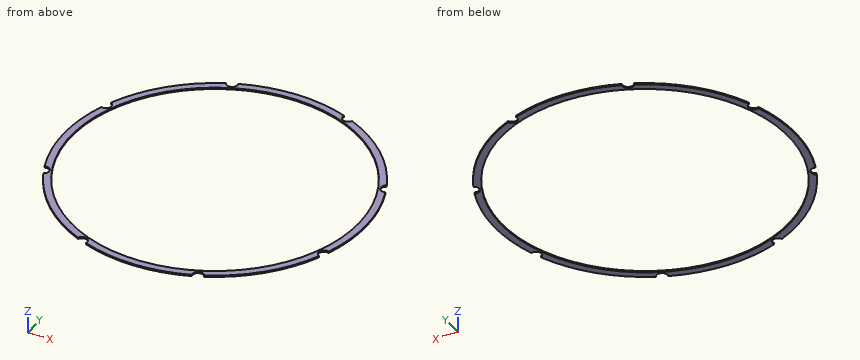
```python
from build123d import *

# Parameters (mm, degrees)
CYLINDER1506_R               = 1.5
CYLINDER1506_DEPTH           = 32
CYLINDER1506_PLACEMENT_ANGLE = 45
CYLINDER1509_R               = 1.5
CYLINDER1509_DEPTH           = 32
CYLINDER1510_R               = 1.5
CYLINDER1510_DEPTH           = 32
CYLINDER1510_PLACEMENT_ANGLE = 135
CYLINDER1511_R               = 1.5
CYLINDER1511_DEPTH           = 32
CYLINDER1508_R               = 1.5
CYLINDER1508_DEPTH           = 32
CYLINDER1508_PLACEMENT_ANGLE = 225
CYLINDER1512_R               = 1.5
CYLINDER1512_DEPTH           = 32
CYLINDER1505_R               = 1.5
CYLINDER1505_DEPTH           = 32
CYLINDER1505_PLACEMENT_ANGLE = 45
CYLINDER1504_R               = 1.5
CYLINDER1504_DEPTH           = 32
COMPOUND1000_PLACEMENT_ANGLE = 22.5
TUBE139_R                    = 42
TUBE139_R_2                  = 40
TUBE139_DEPTH                = 0.4


with BuildPart() as obj1:
    # Cylinder1506 → Cylinder1506 (new body)
    with BuildSketch(Plane.XY):
        Circle(CYLINDER1506_R)
    extrude(amount=CYLINDER1506_DEPTH)


with BuildPart() as obj1_1:
    # Cylinder1506 placement: moved
    add(obj1.part.moved(Location((29.698485, -29.698485, 33.5))).rotate(Axis((29.698485, -29.698485, 33.5), (0, 0, 1)), CYLINDER1506_PLACEMENT_ANGLE))


with BuildPart() as obj2:
    # Cylinder1509 → Cylinder1509 (new body)
    with BuildSketch(Plane(origin=(42, 0, 33.5), x_dir=(0, 1, 0), z_dir=(0, 0, 1))):
        Circle(CYLINDER1509_R)
    extrude(amount=CYLINDER1509_DEPTH)


with BuildPart() as obj3:
    # Cylinder1510 → Cylinder1510 (new body)
    with BuildSketch(Plane.XY):
        Circle(CYLINDER1510_R)
    extrude(amount=CYLINDER1510_DEPTH)


with BuildPart() as obj3_1:
    # Cylinder1510 placement: moved
    add(obj3.part.moved(Location((29.698485, 29.698485, 33.5))).rotate(Axis((29.698485, 29.698485, 33.5), (0, 0, 1)), CYLINDER1510_PLACEMENT_ANGLE))


with BuildPart() as obj4:
    # Cylinder1511 → Cylinder1511 (new body)
    with BuildSketch(Plane(origin=(0, 42, 33.5), x_dir=(-1, 0, 0), z_dir=(0, 0, 1))):
        Circle(CYLINDER1511_R)
    extrude(amount=CYLINDER1511_DEPTH)


with BuildPart() as obj5:
    # Cylinder1508 → Cylinder1508 (new body)
    with BuildSketch(Plane.XY):
        Circle(CYLINDER1508_R)
    extrude(amount=CYLINDER1508_DEPTH)


with BuildPart() as obj5_1:
    # Cylinder1508 placement: moved
    add(obj5.part.moved(Location((-29.698485, 29.698485, 33.5))).rotate(Axis((-29.698485, 29.698485, 33.5), (0, 0, 1)), CYLINDER1508_PLACEMENT_ANGLE))


with BuildPart() as obj6:
    # Cylinder1512 → Cylinder1512 (new body)
    with BuildSketch(Plane(origin=(-42, 0, 33.5), x_dir=(0, -1, 0), z_dir=(0, 0, 1))):
        Circle(CYLINDER1512_R)
    extrude(amount=CYLINDER1512_DEPTH)


with BuildPart() as obj7:
    # Cylinder1505 → Cylinder1505 (new body)
    with BuildSketch(Plane.XY):
        Circle(CYLINDER1505_R)
    extrude(amount=CYLINDER1505_DEPTH)


with BuildPart() as obj7_1:
    # Cylinder1505 placement: moved
    add(obj7.part.moved(Location((-29.698485, -29.698485, 33.5))).rotate(Axis((-29.698485, -29.698485, 33.5), (0, 0, -1)), CYLINDER1505_PLACEMENT_ANGLE))


with BuildPart() as compound1000:
    # Cylinder1504 → Cylinder1504 (new body)
    with BuildSketch(Plane(origin=(0, -42, 33.5), x_dir=(1, 0, 0), z_dir=(0, 0, 1))):
        Circle(CYLINDER1504_R)
    extrude(amount=CYLINDER1504_DEPTH)

    # Compound1000: union obj1, obj2, obj3, obj4, obj5, obj6, obj7
    add(obj1_1.part)
    add(obj2.part)
    add(obj3_1.part)
    add(obj4.part)
    add(obj5_1.part)
    add(obj6.part)
    add(obj7_1.part)


with BuildPart() as compound1000_1:
    # Compound1000 placement: moved
    add(compound1000.part.rotate(Axis((0, 0, 0), (0, 0, 1)), COMPOUND1000_PLACEMENT_ANGLE))


with BuildPart() as cut537:
    # Tube139 → Tube139 (new body)
    with BuildSketch(Plane.XY.offset(38)):
        Circle(TUBE139_R)
        Circle(TUBE139_R_2, mode=Mode.SUBTRACT)
    extrude(amount=TUBE139_DEPTH)

    # Cut537: cut Compound1000
    add(compound1000_1.part, mode=Mode.SUBTRACT)


with BuildPart() as cut537_1:
    # Cut537 placement: moved
    add(cut537.part.moved(Location((0, 0, 1))))


solid = cut537_1.part
```
Here's how the part is built. I have some questions about the finished solid (model axes, mm). Coordinates: 2 decimals unless noted, no trailing zeros. Order: outer loops, then holes, each group sorted by start corner. A loop starts at its lowest first (then second) coordinate and runs counter-clockwise, first axis right, second up.
1) Imagine slicing it at C-C on z = 39.15. List the corners of the cut face in (x, y) for me.
2) Imagine slicing it at A-A on x = 0. List the corners of the cut face in (y, z) for me, and give its area (3 significant figures).
3) I need wall thicknesses on line 1 (Y direction, x = -9, z = 39.35); line 2 (Y direction, x = 4, z = 39.2); line 3 (X direction, y = 8, z = 39.15). Which ranges of each line are inside material? Lowest first, please.
4) Imagine slicing it at B-B on y = -4. List the corners of the cut face in (x, z) for me, and give its area (3 significant figures).
Response values:
1. outline: (-39.35, -14.68) arc R1.5 cw to (-38.2, -17.45) arc R42 ccw to (-17.45, -38.2) arc R1.5 cw to (-14.68, -39.35) arc R42 ccw to (14.68, -39.35) arc R1.5 cw to (17.45, -38.2) arc R42 ccw to (38.2, -17.45) arc R1.5 cw to (39.35, -14.68) arc R42 ccw to (39.35, 14.68) arc R1.5 cw to (38.2, 17.45) arc R42 ccw to (17.45, 38.2) arc R1.5 cw to (14.68, 39.35) arc R42 ccw to (-14.68, 39.35) arc R1.5 cw to (-17.45, 38.2) arc R42 ccw to (-38.2, 17.45) arc R1.5 cw to (-39.35, 14.68) arc R42 ccw to start; hole circle Ø80 at (0, 0)
2. outline: (-42, 39) - (-40, 39) - (-40, 39.4) - (-42, 39.4) - close; (40, 39) - (42, 39) - (42, 39.4) - (40, 39.4) - close
2. area: 1.60 mm2
3. line 1: y = -41.02 to -38.97, 38.97 to 41.02
3. line 2: y = -41.81 to -39.8, 39.8 to 41.81
3. line 3: x = -41.23 to -39.19, 39.19 to 41.23
4. outline: (-41.81, 39) - (-39.8, 39) - (-39.8, 39.4) - (-41.81, 39.4) - close; (39.8, 39) - (41.81, 39) - (41.81, 39.4) - (39.8, 39.4) - close
4. area: 1.61 mm2
